Autodesk Inventor part; units mm, degrees
ref_plane "YZ Plane" through (0, 0, 0) normal (1, 0, 0) x (0, 1, 0)
ref_plane "XZ Plane" through (0, 0, 0) normal (0, 1, 0) x (-1, 0, 0)
ref_plane "XY Plane" through (0, 0, 0) normal (0, 0, 1) x (1, 0, 0)
sketch "Sketch1" plane through (0, 0, 0) normal (0, 0, 1) x (1, 0, 0)
  circle A0 centre (0, 0) radius 112.5
  line L0 (56, 56) -> (-56, 56)
  line L1 (-56, 56) -> (-56, -56)
  line L2 (-56, -56) -> (56, -56)
  line L3 (56, -56) -> (56, 56)
  line L4 (56, 56) -> (-56, -56) construction
  line L5 (-56, 56) -> (56, -56) construction
  dimension "d157" = 225
  dimension "d158" = 112
  dimension "d159" = 112
extrude "Plate5" add sketch "Sketch1" along normal blind 3
sketch "Sketch7" plane through (0, 0, 0) normal (0, 0, -1) x (-1, 0, 0)
  circle A0 centre (0, 80) radius 8.5
  point P0 (0, 0)
  dimension "d160" = 17
  dimension "d161" = 80
extrude "Cut1" cut sketch "Sketch7" against normal blind 3
pattern_circular "Circular Pattern1" count 4 over 360 about axis through (0, 0, -10) along (0, 0, 1) of "Cut1"
chamfer "Corner Chamfer2" distance 33 angle 45 4 edges at (-56, -56, 1.5) (56, -56, 1.5) (-56, 56, 1.5) (56, 56, 1.5)
properties part number "TZS 0972 funnel FLANGE 50-90" material "Stainless Steel"
The listing builds one solid part. Answer for the finished solid, in the listing's coordinates (mm). A direction names the side the tool comes from. Coordinates: 2 decimals unless noted, no trailing zeros. Write each loop counter-clockwise with the first axis right and the second up, starting at its lowest first coordinate (ties: lowest second). Pieces come first, ordered by that corner, then holes. Notation, with made-up numbers: (62.25, 85) - (75.25, 85) arc R22 cw to (75.25, 108) - close; hole circle Ø8 at (19, -7.75). An arc over 180 degrees is marked (long way). Return JSON: item names as keys, results as strings. Group by question number.
1. Which of the six approach directions +Z, -Z, +X, -X, +Y, -Y give full straight-line access (tool end or side, diameter ignored) to faces 5 (the flat face through (-40, 39, 2)), 6 (the flat face through (48, -48, 0))?
2. A cutting plane is placed at B-B, the plane x = 0. Determine the outline of the cut face in (y, z).
3. A cutting plane is placed at A-A, the plane z = 1.85. Determine the outline of the cut face in (x, y).
4. Straight lines are drawn through the part: L1, parallel to Y at x = 0, z = 2.35; L2, parallel to Y at x = 5, z = 1.8; L3, parallel to X at y = 6.5, z = 0.6. For each, find the intervals that lie inside material, in ascending order.
5. Given pin 1 (0.9 mm diameter, centred on x = 9, z = 1.5, fed in from -Y); pin 2 (15.5 mm diameter, centred on x = 0, y = -80, fed in from -Z); pin 3 (0.9 mm diameter, centred on y = 1, z = 1.5, fed in from +X); pin 4 (1.5 mm diameter, centred on y = -62, z = 2.5, fed in from +X), each flat-ended and moving along its own axis, determine where each tip first touches the part or whether it passes through.
6. Determine the mould class of faces 1 (the cylindrical face through (6.745, 74.828, 1.479)), 2 (the flat face through (48, -48, 3)), 3 (the flat face through (-39, -40, 2)), 4 (the cylindrical face through (-112.39, -4.95, 1.48)) for opening direction X: released by +X, released by -X, zero draft, split by the parting line, or undercut.
7. A cutting plane is placed at D-D, the plane x = -41.5. Determine the outline of the cut face in (y, z).
Ans:
{
 "1": {"face 5": "+Z, -Z", "face 6": "-Z, +X, -X, +Y, -Y"},
 "2": {"outline": "(-112.5, 0) - (-88.5, 0) - (-88.5, 3) - (-112.5, 3) - close; (-71.5, 0) - (-56, 0) - (-56, 3) - (-71.5, 3) - close; (56, 0) - (71.5, 0) - (71.5, 3) - (56, 3) - close; (88.5, 0) - (112.5, 0) - (112.5, 3) - (88.5, 3) - close"},
 "3": {"outline": "circle Ø225 at (0, 0); hole circle Ø17 at (-80, 0); hole (-56, -23) - (-23, -56) - (23, -56) - (56, -23) - (56, 23) - (23, 56) - (-23, 56) - (-56, 23) - close; hole circle Ø17 at (0, -80); hole circle Ø17 at (0, 80); hole circle Ø17 at (80, 0)"},
 "4": {"L1": "-112.5 to -88.5, -71.5 to -56, 56 to 71.5, 88.5 to 112.5", "L2": "-112.39 to -86.87, -73.13 to -56, 56 to 73.13, 86.87 to 112.39", "L3": "-112.31 to -85.48, -74.52 to -56, 56 to 74.52, 85.48 to 112.31"},
 "5": {"pin 1": "y = -112.17", "pin 2": "through", "pin 3": "x = 112.5", "pin 4": "x = 94.36"},
 "6": {"face 1": "undercut", "face 2": "zero draft", "face 3": "undercut", "face 4": "split by the parting line"},
 "7": {"outline": "(-104.57, 0) - (-37.5, 0) - (-37.5, 3) - (-104.57, 3) - close; (37.5, 0) - (104.57, 0) - (104.57, 3) - (37.5, 3) - close"}
}
